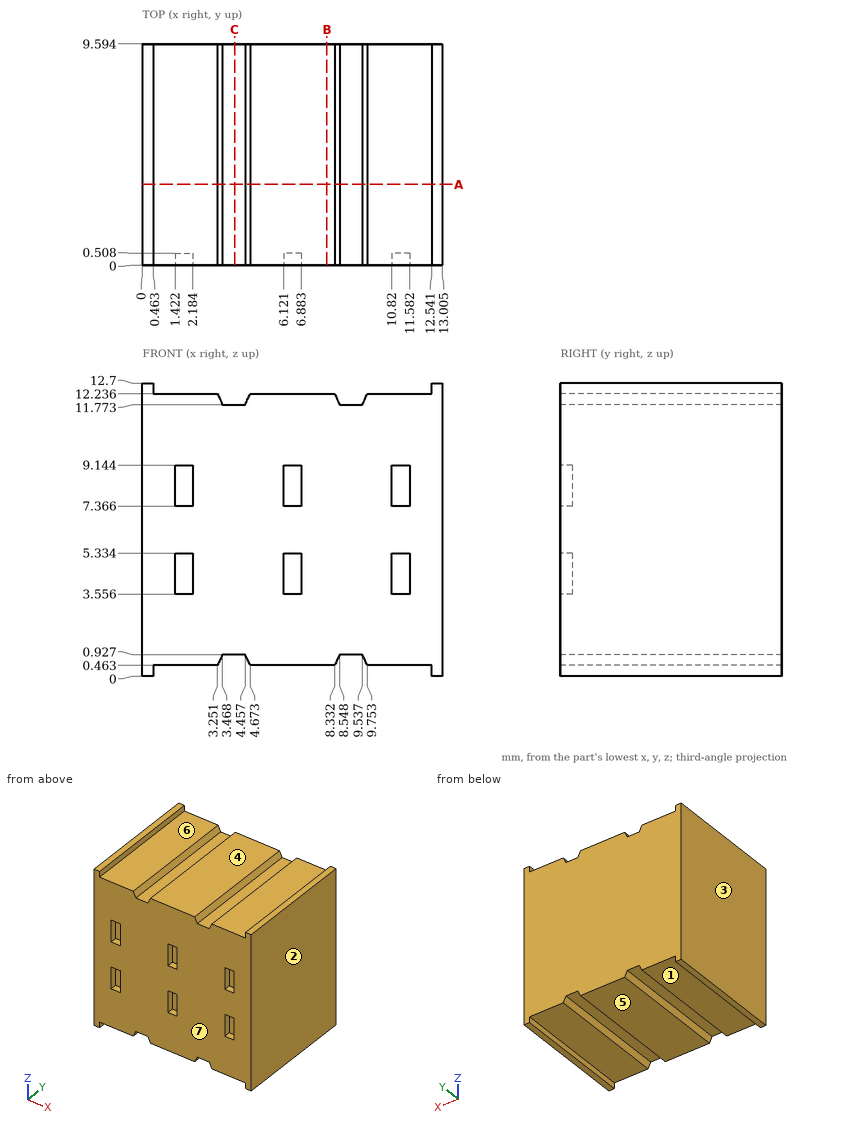
Print and shaded views of the part. All mm, measured from the part's lowest x, y and z. A direction names the side the tool comes from. Round coordinates to 2 decimals unless told otherwise and drop trailing zeros. Order: outer loops, then holes, each group sorted by start corner. A loop starts at its lowest first (then second) coordinate and runs counter-clockwise, first axis right, second up.
Q1. Drop flat-ended pins along their axis: pin 1 (3 mm diameter, centred on x = 2.5, y = 2.5, fed in from +Z); pin 2 (5 mm diameter, centred on x = 3, z = 8.5, fed in from -Y); pin 3 (0.6 mm diameter, centred on x = 1.5, y = 0, fed in from -Z); pin 4 (1.1 mm diameter, centred on x = 4, y = 4.5, fed in from +Z) (1 decimal). Give the stop position or say it passes through.
Q2. Which spindle directions (+Z, -Z, +X, -X, +Y, -Y) get a long thin tool onto all of the face, cutting with end or side? Do the marked faces 5, 6 and 7. Say none if no direction does.
Q3. Slice it at A-A (y = 3.5). Write the cut outline in (x, z) (1 decimal).
Q4. Slice it at C-C (x = 4). Write the cut outline in (y, z), and give its area (3 significant figures).
Q5. Two-plate mould, pull along X, no slides. Class the marked faces 1, 2, 3 and 4: pulls with the +X half, pulls with the -X half, needs draft (parallel to the pull), parting line crosses it, or undercut.
Q6. Slice it at B-B (x = 8). Write the cut outline in (y, z), and give its area (3 significant figures).
Q7. Wall check: L1, parallel to Z at x = 5.75, y = 1.25; L2, parallel to Y at x = 11.25, z = 7.5; L3, parallel to Z at x = 9.5, y = 5.25. Give the ranges that are in metal, low to high.
Results below:
1. pin 1: stops at z = 12.24
1. pin 2: stops at y = 0
1. pin 3: stops at z = 0.46
1. pin 4: stops at z = 12
2. face 5: -Z, +Y, -Y
2. face 6: +Z, +Y, -Y
2. face 7: +Z, -Z, +X, -X, -Y
3. outline: (0, 0) - (0.5, 0) - (0.5, 0.5) - (3.3, 0.5) - (3.5, 0.9) - (4.5, 0.9) - (4.7, 0.5) - (8.3, 0.5) - (8.5, 0.9) - (9.5, 0.9) - (9.8, 0.5) - (12.5, 0.5) - (12.5, 0) - (13, 0) - (13, 12.7) - (12.5, 12.7) - (12.5, 12.2) - (9.8, 12.2) - (9.5, 11.8) - (8.5, 11.8) - (8.3, 12.2) - (4.7, 12.2) - (4.5, 11.8) - (3.5, 11.8) - (3.3, 12.2) - (0.5, 12.2) - (0.5, 12.7) - (0, 12.7) - close
4. outline: (0, 0.93) - (9.59, 0.93) - (9.59, 11.77) - (0, 11.77) - close
4. area: 104 mm2
5. face 1: undercut
5. face 2: pulls with the +X half
5. face 3: pulls with the -X half
5. face 4: undercut
6. outline: (0, 0.46) - (9.59, 0.46) - (9.59, 12.24) - (0, 12.24) - close
6. area: 113 mm2
7. L1: z = 0.46 to 12.24
7. L2: y = 0.51 to 9.59
7. L3: z = 0.93 to 11.77
